Read the model definition and answer for the solid it produces. Units are mm, in the model's axes. A direction names the side the tool comes from. Round coordinates to 2 decimals unless told otherwise and drop trailing zeros. Loops run counter-clockwise (first coordinate to the right, second up) from the corner with the lowest first, then second, coordinate; pieces in that order, holes last. Notation, with made-up numbers: M 60.25,-7.5 L 110.25,-7.5 A26 cw 110.25,27.5 Z; hole C 18.25,71.5 d4. An arc over 180 degrees is marked long. Write each question's results on one line, items separated by ' | '.
```python
from build123d import *

# Parameters (mm, degrees)
SKETCH1_R           = 15
SKETCH1_R_2         = 7.343075537
SKETCH1_R_3         = 7.048050761
SKETCH1_R_4         = 7.405031705
BOSS_EXTRUDE1_DEPTH = 4.7625
SKETCH3_R           = 5
CUT_EXTRUDE1_DEPTH  = 9.525
CUT_EXTRUDE2_DEPTH  = 18.375


with BuildPart() as part:
    # Sketch1 → Boss-Extrude1 (new, symmetric)
    with BuildSketch(Plane.XY):
        with Locations((-135.989964622, 14.806967819)):
            Circle(SKETCH1_R)
        with BuildLine():
            Line((-144.43677034, 2.411344674), (-80.310762347, -41.286331891))
            ThreePointArc((-80.310762347, -41.286331891), (-79.60770007, -28.726487254), (-68.832651313, -35.218198752))
            ThreePointArc((-68.832651313, -35.218198752), (-69.89332652, -39.019804259), (-72.768932333, -41.723159126))
            Line((-72.768932333, -41.723159126), (-49.966216141, -29.780862162))
            ThreePointArc((-49.966216141, -29.780862162), (-59.266125529, -19.888386029), (-46.188084172, -23.53725338))
            ThreePointArc((-46.188084172, -23.53725338), (-46.285689954, -24.706156337), (-46.575803889, -25.842683907))
            Line((-46.575803889, -25.842683907), (4.15447513, 120.715821505))
            ThreePointArc((4.15447513, 120.715821505), (-7.221463009, 117.165978053), (-7.258334859, 129.082856736))
            Line((-7.258334859, 129.082856736), (-144.43677034, 27.202590964))
            ThreePointArc((-144.43677034, 27.202590964), (-128.979332902, 28.06785176), (-120.989964622, 14.806967819))
            ThreePointArc((-120.989964622, 14.806967819), (-128.979332902, 1.546083878), (-144.43677034, 2.411344674))
        make_face()
        with Locations((-76.175726851, -35.218198752)):
            Circle(SKETCH1_R_2)
        with Locations((-53.236134933, -23.53725338)):
            Circle(SKETCH1_R_3)
        with Locations((-2.84319901, 123.138021163)):
            Circle(SKETCH1_R_4)
    extrude(amount=BOSS_EXTRUDE1_DEPTH, both=True)

    # Sketch3 → Cut-Extrude1 (cut)
    with BuildSketch(Plane(origin=(0, 0, -4.7625), x_dir=(-1, 0, 0), z_dir=(0, 0, -1))):
        with Locations((135.989964622, 14.806967819)):
            Circle(SKETCH3_R)
    extrude(amount=-CUT_EXTRUDE1_DEPTH, mode=Mode.SUBTRACT)

    # Sketch5 → Cut-Extrude2 (cut)
    with BuildSketch(Plane(origin=(0, 0, -4.7625), x_dir=(-1, 0, 0), z_dir=(0, 0, -1))):
        Polygon((51.738143119, 70.835792845), (33.841540749, 52.939190474), (49.590550835, 10.464587516), (81.327192371, 12.373558435), (95.883095633, 33.133617185), (93.258260618, 45.303306796), align=None)
    extrude(amount=-CUT_EXTRUDE2_DEPTH, mode=Mode.SUBTRACT)


solid = part.part
```
1. Find section D-D, the plane y = 111.5. Give the vertices of the cut face in (x, z).
Completed:
outline: M -30.93,-4.76 L 0.96,-4.76 L 0.96,4.76 L -30.93,4.76 Z
2. Find section A-A, the plane x = -38. Give the vertices of the cut face in (y, z), then the cut area to 3 significant figures.
Completed:
outline: M -1.07,-4.76 L 41.72,-4.76 L 41.72,4.76 L -1.07,4.76 Z; M 57.1,-4.76 L 106.25,-4.76 L 106.25,4.76 L 57.1,4.76 Z | area: 876 mm2
3. Find section B-B, the plane z = -0.25. Give the vertices of the cut face in (x, y).
Completed:
outline: M -144.44,2.41 L -80.31,-41.29 A7.34 ccw -72.77,-41.72 L -49.97,-29.78 A7.05 ccw -46.58,-25.84 L 4.15,120.72 A7.41 ccw -7.26,129.08 L -144.44,27.2 A15 ccw Z; hole C -135.99,14.81 d10; hole M -95.88,33.13 L -81.33,12.37 L -49.59,10.46 L -33.84,52.94 L -51.74,70.84 L -93.26,45.3 Z
4. Find the intervals of material crossed by L1, parallel to Y at x = -133.5, z = -4; L2, parallel to X at y = 68, z = 0.25; L3, parallel to X at y = 63, z = 0, in increasing order.
Completed:
L1: y = -5.04 to 10.47, 19.14 to 35.33 | L2: x = -89.5 to -56.35, -48.9 to -14.09 | L3: x = -96.24 to -64.48, -43.9 to -15.82
5. Determine the mould class of faces 3 (the face through (1.64, 129.03, 0.07)), 4 (the face through (-61.527, -35.836, 0.067)), 5 (the face through (-41.606, 31.999, -0.067)) for opening direction Y: released by +Y, released by -Y, zero draft, split by the parting line, or undercut.
Completed:
face 3: split by the parting line | face 4: released by -Y | face 5: undercut
6. Find section C-C, the plane x = -134. Give the vertices of the cut face in (y, z).
Completed:
outline: M -4.7,-4.76 L 10.22,-4.76 L 10.22,4.76 L -4.7,4.76 Z; M 19.39,-4.76 L 34.95,-4.76 L 34.95,4.76 L 19.39,4.76 Z
7. Which of the six approach directions +Z, -Z, +X, -X, +Y, -Y give full straight-line access (tool end or side, diameter ignored) to faces 1 (the face through (-65.237, 11.406, -0.067)), 2 (the face through (-21.566, 46.411, 0.067))?
Completed:
face 1: +Z, -Z | face 2: +Z, -Z, +X, -Y
8. Given P1, Ø4, axis at x = -80.5, z = 1, coming from the +Y side; P2, Ø2, axis at x = -17, z = 1.5, coming from the +Y side; P3, Ø2, axis at y = 47.5, z = 1, coming from the -X side, each flat-ended and moving along its own axis, determine where each tip first touches the part or whether it passes through.
Completed:
P1: stops at y = 76.17 | P2: stops at y = 122.59 | P3: stops at x = -118.45
